Source: CAD feature listing. Evaluate the final solid. Frame: model axes, mm. Face numbers are marked on the shaded views. A direction names the side the tool comes from. Give positions to 0.01 mm unless a question says otherwise; leave off trailing zeros. Write each loop counter-clockwise with the first axis right and the second up, starting at its lowest first coordinate (ties: lowest second). Pieces come first, ordered by that corner, then holes.
```python
from build123d import *

# Parameters (mm, degrees)
SKETCH1_R                       = 3.20000000000001
SKETCH1_R_2                     = 3.2000000000000157
SKETCH1_R_3                     = 3.1500000000000266
BOSS_EXTRUDE1_DEPTH             = 9.000000000000002
BOSS_EXTRUDE2_DEPTH             = 6
BOSS_EXTRUDE2_DIRECTION_2_REACH = 245.63
SKETCH3_R                       = 1.3499999999999934
CUT_EXTRUDE1_DEPTH              = 243.3192700509415
CHAMFER1_SIZE                   = 6
CHAMFER1_SIZE_2                 = 10
CHAMFER2_SIZE                   = 5
CHAMFER2_SIZE_2                 = 9
FILLET1_R                       = 2
FILLET2_R                       = 0.5
FILLET3_R                       = 0.5
FILLET4_R                       = 1


with BuildPart() as part:
    # Sketch1 → Boss-Extrude1 (new body)
    with BuildSketch(Plane(origin=(9.000000000000002, 0, 0), x_dir=(0, 0, -1), z_dir=(1, 0, 0))):
        with BuildLine():
            Line((3.5235214674406836, 220.17063085897752), (-29.477274377996263, 239.2218112310119))
            ThreePointArc((-29.477274377996263, 239.2218112310119), (-38.718007493319135, 237.16461837930046), (-37.45821987569468, 227.78186152983258))
            Line((-37.45821987569468, 227.78186152983258), (-25.4578021395881, 217.78186152983255))
            ThreePointArc((-25.4578021395881, 217.78186152983255), (-24.640376533153265, 217.19486094146168), (-23.74722639538112, 216.731139964795))
            Line((-23.74722639538112, 216.731139964795), (-2.7468482860507106, 207.6799595927607))
            ThreePointArc((-2.7468482860507106, 207.6799595927607), (6.279741658038257, 210.96778498862912), (3.5235214674406836, 220.17063085897752))
        make_face()
        with Locations(Location((0.02377470320349104, 214.10830683380283, 0), (0, 0, 180))):
            Circle(SKETCH1_R, mode=Mode.SUBTRACT)
        with Locations(Location((-32.97702114223346, 233.1594872058372, 0), (0, 0, 180))):
            Circle(SKETCH1_R_2, mode=Mode.SUBTRACT)
        with Locations(Location((-20.97660340612688, 223.1594872058372, 0), (0, 0, 180))):
            Circle(SKETCH1_R_3, mode=Mode.SUBTRACT)
    extrude(amount=-BOSS_EXTRUDE1_DEPTH)

    # Sketch2 → Boss-Extrude2 (add)
    with BuildSketch(Plane.ZY):
        Polygon((8.976225296796509, 232.10830683380286), (11.976225296796507, 232.10830683380286), (11.97622529679651, 211.6578287344907), (8.976225296796512, 210.36482624783363), align=None)
    extrude(amount=BOSS_EXTRUDE2_DEPTH)

    # Boss-Extrude2 direction 2: up to this face of the body (flat: up to its plane)
    boss_extrude2_direction_2_end = Plane(part.part.faces().sort_by_distance((9, 223.146004551, 16.682900482))[0])
    # Sketch2 → Boss-Extrude2 direction 2 (add, up to the picked face)
    with BuildSketch(Plane.ZY, mode=Mode.PRIVATE) as boss_extrude2_direction_2_sk1:
        Polygon((8.976225296796509, 232.10830683380286), (11.976225296796507, 232.10830683380286), (11.97622529679651, 211.6578287344907), (8.976225296796512, 210.36482624783363), align=None)
    boss_extrude2_direction_2_tool1 = split(extrude(boss_extrude2_direction_2_sk1.sketch, amount=-BOSS_EXTRUDE2_DIRECTION_2_REACH, mode=Mode.PRIVATE), bisect_by=boss_extrude2_direction_2_end, keep=Keep.BOTH, mode=Mode.PRIVATE)
    add(boss_extrude2_direction_2_tool1.solids().sort_by(Axis((0, 221.556515, 10.460903), (1, 0, 0)))[0])

    # Sketch3 → Cut-Extrude1 (cut, through all)
    with BuildSketch(Plane(origin=(0, 1.43e-15, 8.976225296796544), x_dir=(-1, 0, 0), z_dir=(0, -1.6e-16, -1))):
        with Locations(Location((3, 229.10830683380286, 0), (0, 0, 90))):
            Circle(SKETCH3_R)
    extrude(amount=-CUT_EXTRUDE1_DEPTH, mode=Mode.SUBTRACT)

    # Chamfer1
    # the kernel refuses this chamfer: 10, 6 mm, written as the material it takes off along each edge
    with BuildSketch(Plane(origin=(-6, 221.89433509463086, 35.72677442359438), x_dir=(0.9984760801092615, -0.05067944312803606, 0.021842881995648558), z_dir=(0, -0.3958032841791771, -0.9183353201488973))) as chamfer1_piece_1:
        Polygon((CHAMFER1_SIZE * 0.998476080109, -CHAMFER1_SIZE * 0.0551862070598), (-CHAMFER1_SIZE_2 * 0.0551862070598, -CHAMFER1_SIZE_2 * 0.998476080109), (0, 0), align=None)
    extrude(amount=54.99200253498646, mode=Mode.SUBTRACT)

    # Chamfer2
    # the kernel refuses this chamfer: 9, 5 mm, written as the material it takes off along each edge
    with BuildSketch(Plane(origin=(9.000000000000002, 232.10830683380286, -14.314617746831651), x_dir=(0.060700782983652134, -0.9981560073180803, 0), z_dir=(0, 0, 1))) as chamfer2_piece_1_section:
        Polygon((CHAMFER2_SIZE * 0.998156007318, -CHAMFER2_SIZE * 0.0607007829837), (-CHAMFER2_SIZE_2 * 0.0607007829837, -CHAMFER2_SIZE_2 * 0.998156007318), (0, 0), align=None)
    chamfer2_piece_1 = extrude(amount=49.581686087256315, mode=Mode.PRIVATE)
    chamfer2_piece_1 = split(chamfer2_piece_1, bisect_by=Plane(origin=(5.860742966777749, 228.82016054729928, 11.45934877100172), z_dir=(0, 0.8660462893106784, -0.49996382346246293)), keep=Keep.TOP, mode=Mode.PRIVATE)
    add(chamfer2_piece_1, mode=Mode.SUBTRACT)

    # Fillet1
    fillet1_edges = [part.edges().sort_by_distance(p)[0] for p in [
        (-6, 232.10830683380286, 10.476225296796507),
    ]]
    fillet(fillet1_edges, radius=FILLET1_R)

    # Fillet2
    fillet2_edges = [part.edges().sort_by_distance(p)[0] for p in [
        (4.249475994772133, 227.38666683961173, 8.97622529679651),
    ]]
    fillet(fillet2_edges, radius=FILLET2_R)

    # Fillet3
    fillet3_edges = [part.edges().sort_by_distance(p)[0] for p in [
        (2.6907806455631165, 229.11855056095553, 11.976225296796507),
    ]]
    fillet(fillet3_edges, radius=FILLET3_R)

    # Fillet4
    fillet4_edges = [part.edges().sort_by_distance(p)[0] for p in [
        (0, 219.020091073198, 8.97622529679651),
    ]]
    fillet(fillet4_edges, radius=FILLET4_R)


solid = part.part
```
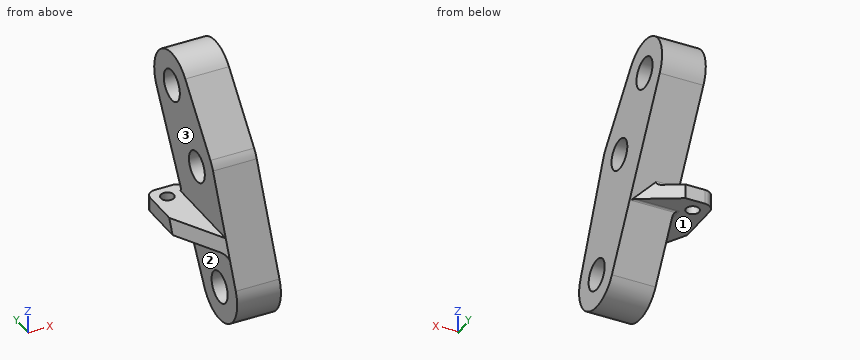
1. Cut plane A-A, the plane z = 20. Return the cut outline in (x, y), then the cut area to 3 significant figures.
2. Cut plane C-C, the plane x = 0.5. Return the cut outline in (y, z).
3. Cut plane B-B, the plane x = -3. Return the cut outline in (y, z), then the cut area to 3 significant figures.
4. Access query for the marked faces 1, 2 and 3. Directions: +Z, -Z, +X, -X, +Y, -Y. A direction counts if a zero-diameter tool reaches every point of the face in a straight line with its end or side. Return the directions, or none.
5. Contact query for flat-ended pins moving along their axis: P1, Ø1.5, axis at x = -1, z = 11, coming from the +Y side; P2, Ø5, axis at y = 213, z = 0.5, coming from the -X side; P3, Ø1, axis at x = 6.5, y = 222, coming from the -Z side. Output: stop coordinate, or through.
6. Cut plane D-D, the plane z = 10. Return the cut outline in (x, y), then the cut area to 3 significant figures.
7. Line query: L1, parallel to X at y = 215, z = -4; L2, parallel to Z at x = -1.5, y = 226.5; L3, parallel to Z at x = 4.75, y = 216. Output: solid intervals per line, ascending.
Response values:
1. outline: (0, 215.12) - (9, 215.12) - (9, 220.16) - (0, 220.16) - close; (0, 226.15) - (9, 226.15) - (9, 233.75) - (0, 233.75) - close
1. area: 114 mm2
2. outline: (207.68, 2.75) arc R7 ccw to (220.17, -3.52) - (227.24, 8.73) arc R0.5 cw to (227.68, 8.98) - (231.83, 8.98) - (231.83, 11.98) - (229.98, 11.98) arc R0.5 cw to (229.55, 12.73) - (239.22, 29.48) arc R7 ccw to (227.78, 37.46) - (217.78, 25.46) arc R7 ccw to (216.73, 23.75) - close; hole circle Ø6.4 at (214.11, -0.02); hole circle Ø6.3 at (223.16, 20.98); hole circle Ø6.4 at (233.16, 32.98)
3. outline: (215.81, 8.98) - (227.76, 8.98) - (227.76, 11.98) - (217.1, 11.98) - close; (230.46, 8.98) - (232.11, 8.98) - (232.11, 11.98) - (230.46, 11.98) - close
3. area: 38.9 mm2
4. face 1: -Z, -X, +Y
4. face 2: -Z, -X, +Y, -Y
4. face 3: +Z, -X, +Y, -Y
5. P1: stops at y = 232.11
5. P2: stops at x = 0
5. P3: stops at z = -1.22
6. outline: (-6, 221.7) - (0, 210.81) - (9, 210.81) - (9, 227.98) - (7.44, 227.98) - (0, 232.11) - (-4, 232.11) arc R2 ccw to (-6, 230.11) - close; hole circle Ø2.7 at (-3, 229.11)
6. area: 258 mm2
7. L1: x = 0 to 9
7. L2: z = 8.98 to 11.98
7. L3: z = -6.76 to -2.6, 2.56 to 22.05
